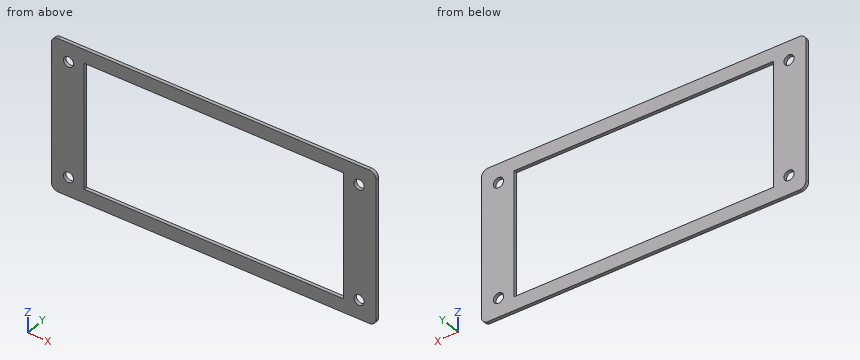
Autodesk Inventor part; units mm, degrees
ref_plane "YZ Plane" through (0, 0, 0) normal (1, 0, 0) x (0, 1, 0)
ref_plane "XZ Plane" through (0, 0, 0) normal (0, 1, 0) x (-1, 0, 0)
ref_plane "XY Plane" through (0, 0, 0) normal (0, 0, 1) x (1, 0, 0)
sketch "Эскиз1" plane through (0, 0, 0) normal (0, 1, 0) x (-1, 0, 0)
  line L0 (0, 0) -> (75.2, 0)
  line L1 (75.2, 0) -> (75.2, 36.7)
  line L2 (75.2, 36.7) -> (0, 36.7)
  line L3 (0, 36.7) -> (0, 0)
  line L4 (0, 0) -> (-10, 0)
  line L5 (-10, 0) -> (-10, -4)
  line L6 (-10, -4) -> (0, -4)
  line L7 (0, -4) -> (0, 0)
  line L8 (-10, -4) -> (85.2, -4)
  line L9 (85.2, -4) -> (85.2, 40.7)
  line L10 (85.2, 40.7) -> (-10, 40.7)
  line L11 (-10, 40.7) -> (-10, -4)
  line L12 (75.2, 36.7) -> (80.2, 36.7)
  line L13 (80.2, 36.7) -> (80.2, 0)
  line L14 (80.2, 0) -> (80.2, 36.7)
  line L15 (80.2, 36.7) -> (80.2, 35.15)
  line L16 (80.2, 0) -> (80.2, 1.55)
  line L17 (0, 0) -> (-5, 0)
  line L18 (-5, 0) -> (-5, 1.55)
  line L19 (-5, 1.55) -> (-5, 36.7)
  line L20 (-5, 36.7) -> (-5, 35.15)
  circle A0 centre (-5, 35.15) radius 1.5
  circle A1 centre (-5, 1.55) radius 1.5
  circle A2 centre (80.2, 35.15) radius 1.5
  circle A3 centre (80.2, 1.55) radius 1.5
  dimension "d0" = 75.2
  dimension "d1" = 36.7
  dimension "d2" = 10
  dimension "d3" = 4
  dimension "d4" = 95.2
  dimension "d5" = 44.7
  dimension "d6" = 5
  dimension "d7" = 1.55
  dimension "d8" = 1.55
  dimension "d9" = 5
  dimension "d10" = 1.55
  dimension "d11" = 1.55
  dimension "d12" = 3
  dimension "d13" = 3
  dimension "d14" = 3
  dimension "d15" = 3
extrude "Выдавливание1" add sketch "Эскиз1" along normal blind 1
fillet "Сопряжение1" radius 2 4 edges at (-85.2, 0.5, 40.7) (-85.2, 0.5, -4) (10, 0.5, -4) (10, 0.5, 40.7)
sketch "Эскиз2" plane through (0, 1, 0) normal (0, 1, 0) x (1, 0, 0)
  line L0 (0, 0) -> (0.4, 0)
  line L1 (0.4, 0) -> (-75.6, 0)
  line L2 (-75.6, 0) -> (-75.6, -36.7)
  line L3 (-75.6, -36.7) -> (0.4, -36.7)
  line L4 (0.4, -36.7) -> (0.4, 0)
  dimension "d19" = 0.4
  dimension "d20" = 76
extrude "Выдавливание2" cut sketch "Эскиз2" against normal blind 10
properties part number "metal_holder" material "Серебро"
Source: CAD feature listing. Evaluate the final solid. Frame: model axes, mm. Give positions to 0.01 mm unless a question says otherwise; leave off trailing zeros. Write each loop counter-clockwise with the first axis right and the second up, starting at its lowest first coordinate (ties: lowest second). Pieces come first, ordered by that corner, then holes.
1. Section query C-C (y = 0.8). Return the cut outline in (x, z), then the cut area to 3 significant figures.
2. Section query B-B (x = -80.2). Return the cut outline in (y, z), then the cut area to 3 significant figures.
3. Material intervals for line 1 along Z through (x, y) = (-80.2, 0.85); line 2 along X through (y, z) = (0.75, 35.15); line 3 along Z through (x, y) = (-67.5, 0.2), sorted ascending.
4. Section query A-A (z = 30). Return the cut outline in (x, y).
5. Section query D-D (x = -6). Return the cut outline in (y, z).
Output values:
1. outline: (-85.2, -2) arc R2 ccw to (-83.2, -4) - (8, -4) arc R2 ccw to (10, -2) - (10, 38.7) arc R2 ccw to (8, 40.7) - (-83.2, 40.7) arc R2 ccw to (-85.2, 38.7) - close; hole circle Ø3 at (-80.2, 1.55); hole circle Ø3 at (-80.2, 35.15); hole (-75.6, 0) - (0.4, 0) - (0.4, 36.7) - (-75.6, 36.7) - close; hole circle Ø3 at (5, 1.55); hole circle Ø3 at (5, 35.15)
1. area: 1,430 mm2
2. outline: (0, -4) - (1, -4) - (1, 0.05) - (0, 0.05) - close; (0, 3.05) - (1, 3.05) - (1, 33.65) - (0, 33.65) - close; (0, 36.65) - (1, 36.65) - (1, 40.7) - (0, 40.7) - close
2. area: 38.7 mm2
3. line 1: z = -4 to 0.05, 3.05 to 33.65, 36.65 to 40.7
3. line 2: x = -85.2 to -81.7, -78.7 to -75.6, 0.4 to 3.5, 6.5 to 10
3. line 3: z = -4 to 0, 36.7 to 40.7
4. outline: (-85.2, 0) - (-75.6, 0) - (-75.6, 1) - (-85.2, 1) - close; (0.4, 0) - (10, 0) - (10, 1) - (0.4, 1) - close
5. outline: (0, -4) - (1, -4) - (1, 0) - (0, 0) - close; (0, 36.7) - (1, 36.7) - (1, 40.7) - (0, 40.7) - close
